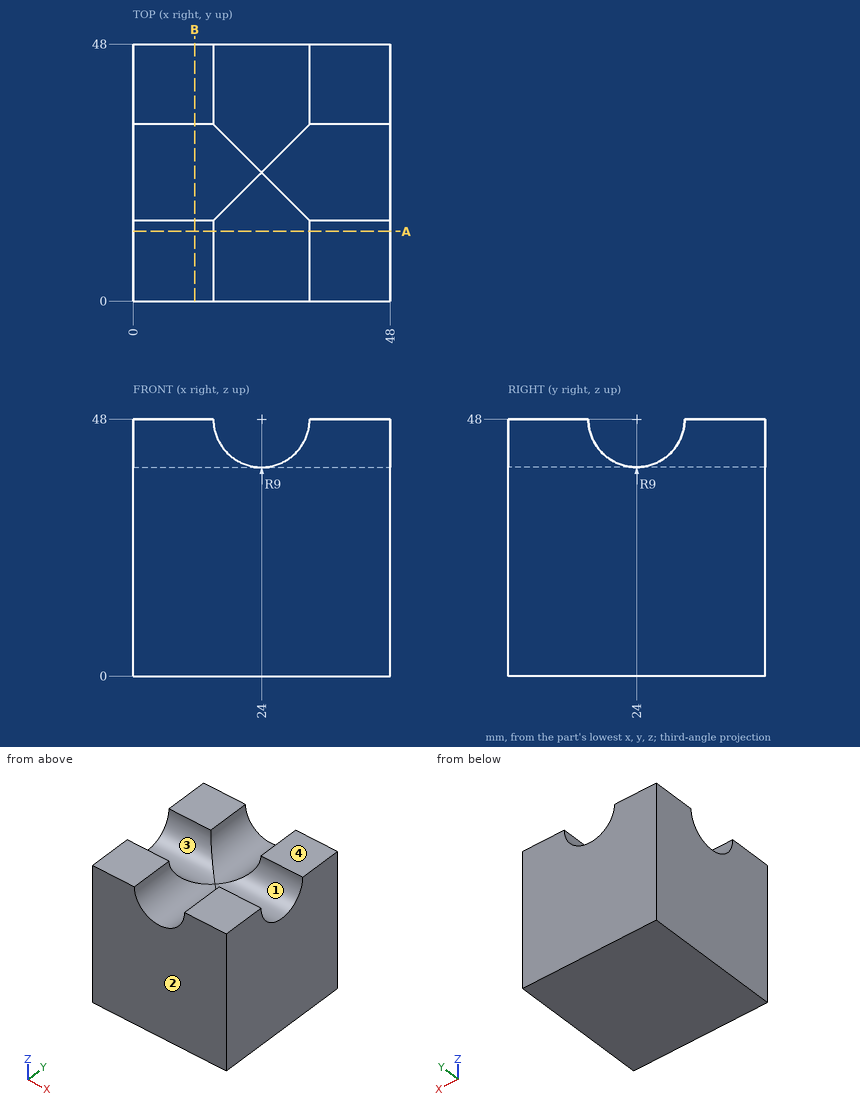
Could you check a few things on this drawing? It's one solid part, dimensions in mm from its lowest x, y, z. Give positions to 0.01 mm unless a question says otherwise; leave off trailing zeros. Write each loop counter-clockwise with the first axis right and the second up, starting at its lowest first coordinate (ties: lowest second). Pieces come first, ordered by that corner, then holes. Notation, with made-up numbers: (-2, -3) - (52, -3) arc R22 cw to (52, 22) - close; hole circle Ø4 at (58.25, -23.5). An arc over 180 degrees is marked (long way). Use CSV: the item, a comma, the result in double quotes. Start each with the question number.
Item 1: If I drill on line 1 along Z through (x, y) = (35.5, 24.5); line 2 along Y through (x, z) = (41, 41); line 3 along Z through (x, y) = (29, 40.5), over which ranges is the centre line in solid material (lowest first)?
Item 2: If we mould it in two halves opening along Y, with no side actions, what happens to the marked faces 1, 2, 3 and 4? For each: pulls with the +Y half, pulls with the -Y half, needs draft (parallel to the pull), parting line crosses it, or undercut.
Item 3: I want a section at A-A, the plane y = 13. Please give me the cut outline in (x, z).
Item 4: I'm going to push a flat-ended pin straight in: pin 1 (8 mm diameter, centred on x = 17.5, y = 20.5, fed in from +Z). Where does the tip first touch, or does it pass through?
Findings:
1,line 1,"z = 0 to 39.01"
1,line 2,"y = 0 to 18.34, 29.66 to 48"
1,line 3,"z = 0 to 40.52"
2,face 1,"undercut"
2,face 2,"pulls with the -Y half"
2,face 3,"undercut"
2,face 4,"needs draft"
3,outline,"(0, 0) - (48, 0) - (48, 48) - (33, 48) arc R9 cw to (15, 48) - (0, 48) - close"
4,pin 1,"stops at z = 42.87"
